```python
from build123d import *

# Parameters (mm, degrees)
F1_W     = 80
F1_H     = 48.65
F2_DEPTH = 3.175
F3_W     = 15
F3_H     = 3.175
F4_DEPTH = 3.175
F5_W     = 3.175
F5_H     = 15
F6_DEPTH = 3.176
F7_R     = 2.05
F8_DEPTH = 3.176


with BuildPart() as f2:
    # F1 (on Top) → F2 (new body)
    with BuildSketch(Plane.XY):
        Rectangle(F1_W, F1_H)
    extrude(amount=F2_DEPTH)

    # F3 (on face) → F4 (join, through all)
    with BuildSketch(Plane.XY.offset(3.175)):
        with Locations((-17.5, -25.9125)):
            Rectangle(F3_W, F3_H)
        with Locations((17.5, -25.9125)):
            Rectangle(F3_W, F3_H)
        with Locations((-17.5, 25.9125)):
            Rectangle(F3_W, F3_H)
        with Locations((17.5, 25.9125)):
            Rectangle(F3_W, F3_H)
    extrude(amount=-F4_DEPTH)

    # F5 (on face) → F6 (cut, through all)
    with BuildSketch(Plane.XY.offset(3.175)):
        with Locations((38.4125, 0)):
            Rectangle(F5_W, F5_H)
        with Locations((-38.4125, 0)):
            Rectangle(F5_W, F5_H)
    extrude(amount=-F6_DEPTH, mode=Mode.SUBTRACT)

    # F7 (on face) → F8 (cut, through all)
    with BuildSketch(Plane.XY.offset(3.175)):
        with Locations((11.6, 18)):
            Circle(F7_R)
        with Locations((21, 18)):
            Circle(F7_R)
        with Locations((21, -18)):
            Circle(F7_R)
        with Locations((11.6, -18)):
            Circle(F7_R)
    extrude(amount=-F8_DEPTH, mode=Mode.SUBTRACT)


solid = f2.part
```
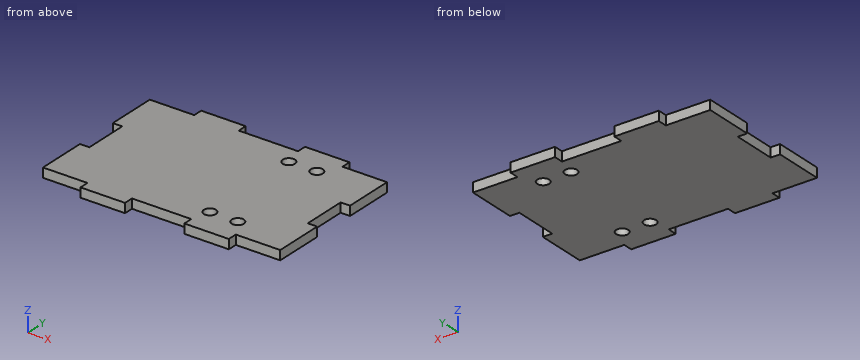
Verification items for the finished model (mm, model axes). Give positions to 0.01 mm unless a question says otherwise; leave off trailing zeros. Order: outer loops, then holes, each group sorted by start corner. A loop starts at its lowest first (then second) coordinate and runs counter-clockwise, first axis right, second up. Notation, with made-up numbers: M 19,49 L 73,49 A10 cw 73,68 Z; hole C 76.5,-16 d2. An arc over 180 degrees is marked long. Return JSON: item names as keys, results as strings. Group by question number.
1) Section check C-C on z = 0.75. Give the number of separate pieces and of enclosed holes in the cut face, and give its area (3 significant figures).
2) Section check D-D on y = -3.5. Record the cut outline in (x, z) (3 decimals), and give its area (3 significant figures).
3) Section check A-A on x = 21. Record the cut outline in (y, z) (3 decimals), and give its area (3 significant figures).
4) Section check B-B on y = -18. Record the cut outline in (x, z) (3 decimals), and give its area (3 significant figures).
5) Scan lines: line 1 (Y direction, x = 11.6, z = 1); line 2 (Y direction, x = 1, z = 0.6) (3 decimals); line 3 (X direction, y = 6.5, z = 2) (3 decimals). Record each from-to range of solid material in increasing order.
6) Go/stop test with flat-tipped pins: pin 1 Ø1 at (x, z) = (-2.5, 1.5) entering from -Y (3 decimals); pin 2 Ø1 at (x, z) = (-8, 2.5) entering from +Y (3 decimals); pin 3 Ø1 at (y, z) = (3.5, 1) entering from +X (3 decimals); pin 4 Ø3.5 at (x, y) = (11.6, -18) entering from +Z. Record where each tip stops, or that it passes through.
Answer block:
{
 "1": {"separate pieces": "1", "enclosed holes": "4", "area": "3,930 mm^2"},
 "2": {"outline": "M -36.825,0 L 36.825,0 L 36.825,3.175 L -36.825,3.175 Z", "area": "234 mm^2"},
 "3": {"outline": "M -27.5,0 L -20.05,0 L -20.05,3.175 L -27.5,3.175 Z; M -15.95,0 L 15.95,0 L 15.95,3.175 L -15.95,3.175 Z; M 20.05,0 L 27.5,0 L 27.5,3.175 L 20.05,3.175 Z", "area": "149 mm^2"},
 "4": {"outline": "M -40,0 L 9.55,0 L 9.55,3.175 L -40,3.175 Z; M 13.65,0 L 18.95,0 L 18.95,3.175 L 13.65,3.175 Z; M 23.05,0 L 40,0 L 40,3.175 L 23.05,3.175 Z", "area": "228 mm^2"},
 "5": {"line 1": "y = -27.5 to -20.05, -15.95 to 15.95, 20.05 to 27.5", "line 2": "y = -24.325 to 24.325", "line 3": "x = -36.825 to 36.825"},
 "6": {"pin 1": "stops at y = -24.325", "pin 2": "stops at y = 24.325", "pin 3": "stops at x = 36.825", "pin 4": "passes through"}
}
